Autodesk Inventor part; units mm, degrees
ref_plane "YZ Plane" through (0, 0, 0) normal (1, 0, 0) x (0, 1, 0)
ref_plane "XZ Plane" through (0, 0, 0) normal (0, 1, 0) x (-1, 0, 0)
ref_plane "XY Plane" through (0, 0, 0) normal (0, 0, 1) x (1, 0, 0)
sketch "Sketch2" plane through (0, 0, 0) normal (0, 1, 0) x (-1, 0, 0)
  circle A0 centre (-33.79, -5.085) radius 2
  circle A1 centre (-33.79, 5.085) radius 2
  circle A2 centre (13.47, -5.085) radius 2
  circle A3 centre (13.47, 5.085) radius 2
  line L0 (20, 15) -> (-45, 15)
  line L1 (-45, 15) -> (-45, -15)
  line L2 (-45, -15) -> (20, -15)
  line L3 (20, -15) -> (20, 15)
  line L4 (20, 30) -> (0, 30)
  line L5 (0, -30) -> (20, -30)
  line L6 (20, -30) -> (20, 30)
  circle A4 centre (14, 24) radius 2
  circle A5 centre (14, -24) radius 2
  line L7 (0, 30) -> (0, 15)
  line L8 (0, -30) -> (0, -15)
  line L9 (9.66, 9.91) -> (-30.22, 9.91)
  line L10 (-30.22, 9.91) -> (-30.22, -9.91)
  line L11 (-30.22, -9.91) -> (9.66, -9.91)
  line L12 (9.66, -9.91) -> (9.66, 9.91)
  point P0 (0, 0)
  dimension "d27" = 4
  dimension "d28" = 4
  dimension "d29" = 4
  dimension "d30" = 4
  dimension "d31" = 13.47
  dimension "d32" = 5.085
  dimension "d33" = 10.17
  dimension "d34" = 13.47
  dimension "d35" = 33.79
  dimension "d36" = 5.085
  dimension "d37" = 10.17
  dimension "d38" = 33.79
  dimension "d39" = 30
  dimension "d40" = 65
  dimension "d41" = 20
  dimension "d42" = 15
  dimension "d43" = 60
  dimension "d44" = 30
  dimension "d45" = 20
  dimension "d46" = 4
  dimension "d47" = 4
  dimension "d48" = 6
  dimension "d49" = 6
  dimension "d50" = 6
  dimension "d51" = 6
  dimension "d52" = 9.66
  dimension "d53" = 19.82
  dimension "d54" = 9.91
  dimension "d55" = 39.88
extrude "Extrusion2" add sketch "Sketch2" along normal blind 3.18
chamfer "Chamfer1" distance 10 angle 45 1 edges at (0, 1.59, -30)
chamfer "Chamfer2" distance 10 angle 45 1 edges at (0, 1.59, 30)
properties part number "Pinza_sostenedor"
Build history of the part. All positions in model axes, mm. A direction names the side the tool comes from. Round coordinates to 2 decimals unless told otherwise and drop trailing zeros. Write each loop counter-clockwise with the first axis right and the second up, starting at its lowest first coordinate (ties: lowest second). Pieces come first, ordered by that corner, then holes. Notation, with made-up numbers: M 70.5,30 L 99.5,30 A31 ccw 99.5,62 Z; hole C 18.5,81.25 d10. An arc over 180 degrees is marked long. Answer as a JSON object with one key per item and string values. Group by question number.
(1) Cut at D-D (z = 6). Give the cut face in (x, y).
(2) Cut at B-B (x = 10). Give the cut face in (y, z), and give its area (3 significant figures).
(3) Which spindle directions (+Z, -Z, +X, -X, +Y, -Y) get a long thin tool onto all of the face, cutting with end or side? Do faces 1 (the flat face through (23, 2, -15)), 2 (the flat face through (30.22, 2, 0)), 3 (the flat face through (22, 2, 15)). Say none if no direction does.
(4) Cut at A-A (z = 24). Give the cut face in (x, y), and give its area (3 significant figures).
(5) Cut at C-C (y = 2.4). Give the cut face in (x, z) (3 decimals), and give its area (3 significant figures).
(6) Drill centre lines: L1, parallel to X at y = 1.3, z = 5; L2, parallel to Z at x = 33.79, y = 1.95 (3 decimals); L3, parallel to Z at x = 6.5, y = 2. Where is each one in solid material? Low to high.
(7) Flat gauge pins, fed straight in: pin 1 (2.5 mm diameter, centred on x = 33.79, z = -5.085, fed in from +Y); pin 2 (1.6 mm diameter, centred on x = 19, y = 2, fed in from -Z); pin 3 (1.6 mm diameter, centred on x = 9, y = 2, fed in from +Z). Where does each tip first touch, or does it go through?
Responses:
{
 "1": {"outline": "M -20,0 L -15.25,0 L -15.25,3.18 L -20,3.18 Z; M -11.69,0 L -9.66,0 L -9.66,3.18 L -11.69,3.18 Z; M 30.22,0 L 32.01,0 L 32.01,3.18 L 30.22,3.18 Z; M 35.57,0 L 45,0 L 45,3.18 L 35.57,3.18 Z"},
 "2": {"outline": "M 0,-15 L 3.18,-15 L 3.18,-9.91 L 0,-9.91 Z; M 0,9.91 L 3.18,9.91 L 3.18,15 L 0,15 Z", "area": "32.4 mm2"},
 "3": {"face 1": "-Z, +X, +Y, -Y", "face 2": "+Y, -Y", "face 3": "+Z, +X, +Y, -Y"},
 "4": {"outline": "M -20,0 L -16,0 L -16,3.18 L -20,3.18 Z; M -12,0 L -4,0 L -4,3.18 L -12,3.18 Z", "area": "38.2 mm2"},
 "5": {"outline": "M -20,-30 L -10,-30 L 0,-20 L 0,-15 L 45,-15 L 45,15 L 0,15 L 0,20 L -10,30 L -20,30 Z; hole C -14,-24 d4; hole C -14,24 d4; hole C -13.47,-5.085 d4; hole C -13.47,5.085 d4; hole M -9.66,-9.91 L 30.22,-9.91 L 30.22,9.91 L -9.66,9.91 Z; hole C 33.79,-5.085 d4; hole C 33.79,5.085 d4", "area": "1,580 mm2"},
 "6": {"L1": "x = -20 to -15.47, -11.47 to -9.66, 30.22 to 31.79, 35.79 to 45", "L2": "z = -15 to -7.085, -3.085 to 3.085, 7.085 to 15", "L3": "z = -15 to -9.91, 9.91 to 15"},
 "7": {"pin 1": "passes through", "pin 2": "stops at z = -15", "pin 3": "stops at z = 15"}
}
